from build123d import *

# Parameters (mm, degrees)
SKETCH1_W               = 31.5
SKETCH1_H               = 60
BOSS_EXTRUDE1_DEPTH     = 12.5
SKETCH2_W               = 5.015
SKETCH2_H               = 40.03
SKETCH2_W_2             = 10
CUT_EXTRUDE1_DEPTH      = 13.765
SKETCH6_R               = 3.25
CUT_EXTRUDE2_DEPTH      = 12
BOSS_EXTRUDE5_DEPTH     = 31.5
BOSS_EXTRUDE6_DEPTH     = 2
CUT_EXTRUDE3_DEPTH      = 61.634148794
CUT_EXTRUDE3_DEPTH_BACK = 61.634148794
SKETCH10_R              = 1.6


with BuildPart() as part:
    # Sketch1 → Boss-Extrude1 (new, symmetric)
    with BuildSketch(Plane(origin=(0, 0, 0), x_dir=(0, 0, -1), z_dir=(1, 0, 0))):
        with Locations((15.75, 20)):
            Rectangle(SKETCH1_W, SKETCH1_H)
    extrude(amount=BOSS_EXTRUDE1_DEPTH, both=True)

    # Sketch2 → Cut-Extrude1 (cut, symmetric)
    with BuildSketch(Plane(origin=(0, 0, -31.5), x_dir=(-1, 0, 0), z_dir=(0, 0, -1))):
        with Locations((7.5075, 20)):
            Rectangle(SKETCH2_W, SKETCH2_H)
        with Locations((0, 20)):
            Rectangle(SKETCH2_W_2, SKETCH2_H)
        with Locations((-7.5075, 20)):
            Rectangle(SKETCH2_W, SKETCH2_H)
    extrude(amount=CUT_EXTRUDE1_DEPTH, both=True, mode=Mode.SUBTRACT)

    # Sketch6 → Cut-Extrude2 (cut)
    with BuildSketch(Plane(origin=(0, 0, -31.5), x_dir=(-1, 0, 0), z_dir=(0, 0, -1))):
        with Locations(Location((-5, 44, 0), (0, 0, 90))):
            Circle(SKETCH6_R)
        with Locations(Location((5, 44, 0), (0, 0, 90))):
            Circle(SKETCH6_R)
        with Locations(Location((5, -4, 0), (0, 0, 90))):
            Circle(SKETCH6_R)
        with Locations(Location((-5, -4, 0), (0, 0, 90))):
            Circle(SKETCH6_R)
    extrude(amount=-CUT_EXTRUDE2_DEPTH, mode=Mode.SUBTRACT)

    # Sketch9 → Boss-Extrude5 (add)
    with BuildSketch(Plane(origin=(0, 0, -31.5), x_dir=(-1, 0, 0), z_dir=(0, 0, -1))):
        with BuildLine():
            Line((11.949417382, -20.681826368), (11.949417382, -24.669417382))
            Line((11.949417382, -24.669417382), (17.5, -24.669417382))
            Line((17.5, -24.669417382), (17.5, -10))
            Line((17.5, -10), (8.113106842, -10))
            ThreePointArc((8.113106842, -10), (13.410384211, -14.127322804), (11.949417382, -20.681826368))
        make_face()
        with BuildLine():
            Line((-17.5, -24.669417382), (-11.949417382, -24.669417382))
            Line((-11.949417382, -24.669417382), (-11.949417382, -20.681826368))
            ThreePointArc((-11.949417382, -20.681826368), (-13.410384211, -14.127322804), (-8.113106842, -10))
            Line((-8.113106842, -10), (-17.5, -10))
            Line((-17.5, -10), (-17.5, -24.669417382))
        make_face()
    extrude(amount=-BOSS_EXTRUDE5_DEPTH)

    # Sketch9<4> → Boss-Extrude6 (add)
    with BuildSketch(Plane(origin=(0, 0, -31.5), x_dir=(-1, 0, 0), z_dir=(0, 0, -1))):
        with BuildLine():
            Line((8.113106842, -10), (-8.113106842, -10))
            ThreePointArc((-8.113106842, -10), (-13.410384211, -14.127322804), (-11.949417382, -20.681826368))
            Line((-11.949417382, -20.681826368), (-11.949417382, -24.669417382))
            Line((-11.949417382, -24.669417382), (11.949417382, -24.669417382))
            Line((11.949417382, -24.669417382), (11.949417382, -20.681826368))
            ThreePointArc((11.949417382, -20.681826368), (13.410384211, -14.127322804), (8.113106842, -10))
        make_face()
    extrude(amount=-BOSS_EXTRUDE6_DEPTH)

    # Sketch10 → Cut-Extrude3 (cut, two sides: drawn at the far end of the back side and taken through both)
    with BuildSketch(Plane.XY.offset(-29.5).offset(-CUT_EXTRUDE3_DEPTH_BACK)):
        with Locations((-7.5, -16.25)):
            Circle(SKETCH10_R)
        with Locations((7.5, -16.25)):
            Circle(SKETCH10_R)
    extrude(amount=CUT_EXTRUDE3_DEPTH + CUT_EXTRUDE3_DEPTH_BACK, mode=Mode.SUBTRACT)


solid = part.part
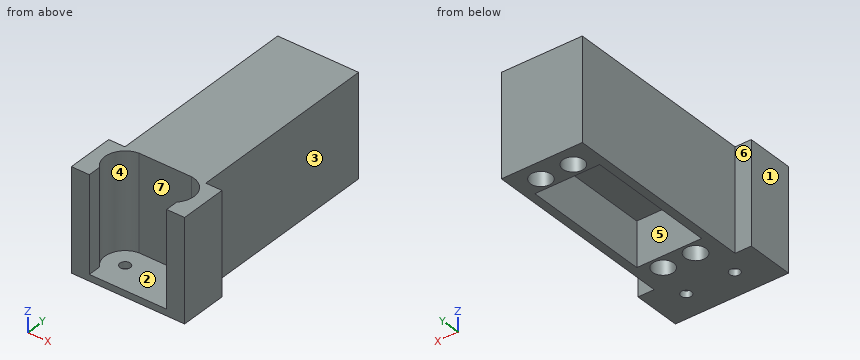
Verification items for the finished model (mm, model axes). Face numbers are marked on the shaded views. A direction names the side the tool comes from. Give positions to 0.01 mm unless a question says otherwise; leave off trailing zeros. Write each loop counter-clockwise with the first axis right and the second up, starting at its lowest first coordinate (ties: lowest second). Pieces come first, ordered by that corner, then holes. Notation, with made-up numbers: M -9,-31 L 36,-31 A23 cw 36,7 Z; hole C -28,-33.5 d8. An arc over 180 degrees is marked long. Use CSV: the item, a comma, the result in double quotes.
1) Release check for a two-part mould opening along X. For the marked faces 1, 2 and 3 record: released by +X, released by -X, zero draft, split by the parting line, or undercut.
Final values:
face 1,"released by -X"
face 2,"undercut"
face 3,"released by +X"
2) Go/stop test with flat-tipped pins: pin 1 Ø3 at (x, z) = (-7, -10) entering from -Y; pin 2 Ø8 at (y, z) = (39, -22.5) entering from +X; pin 3 Ø2.5 at (x, z) = (-16, -14.5) entering from +Y; pin 4 Ø2.5 at (x, y) = (7.5, -16.25) entering from +Z. Record where each tip stops, or that it passes through.
Final values:
pin 1,"y = -10.05"
pin 2,"x = 12.5"
pin 3,"y = -10"
pin 4,"through"
3) Cross-section at C-C (x = 5). Enter the section's corners in (y, z) (3 decimals), plus the area to 3 significant figures.
Final values:
outline,"M -24.669,-31.5 L -7.25,-31.5 L -7.25,-19.5 L -0.75,-19.5 L -0.75,-31.5 L -0.015,-31.5 L -0.015,-17.735 L 40.015,-17.735 L 40.015,-31.5 L 40.75,-31.5 L 40.75,-19.5 L 47.25,-19.5 L 47.25,-31.5 L 50,-31.5 L 50,0 L -10,0 L -10,-29.5 L -24.669,-29.5 Z"
area,"1,210 mm²"
4) Cross-section at B-B (y = -16.25). Enter the section's corners in (x, z), plus the area to 3 significant figures.
Final values:
outline,"M -17.5,-31.5 L -9.1,-31.5 L -9.1,-29.5 L -13.78,-29.5 L -13.78,0 L -17.5,0 Z; M -5.9,-31.5 L 5.9,-31.5 L 5.9,-29.5 L -5.9,-29.5 Z; M 9.1,-31.5 L 17.5,-31.5 L 17.5,0 L 13.78,0 L 13.78,-29.5 L 9.1,-29.5 Z"
area,"277 mm²"
5) Material ranges on line 1 along X through (y, z) = (44, -23); line 2 along X through (y, z) = (20.5, -23) (3 decimals); line 3 along Y through (x, z) = (15.5, -15.5), recorded low to high.
Final values:
line 1,"-12.5 to -8.25, -1.75 to 1.75, 8.25 to 12.5"
line 2,"-12.5 to -10.015, 10.015 to 12.5"
line 3,"-24.67 to -10"
6) Access from +Z, -Z, +X, -X, +Y, -Y to the whole of each face (thin tool, end or side, straight path). Record for the marked faces 4, 5, 6 and 7.
Final values:
face 4,"+Z"
face 5,"-Z"
face 6,"+Z, -Z, -X, +Y"
face 7,"+Z, -Y"
7) Cross-section at D-D (y = 26.5). Enter the section's corners in (x, z) (3 decimals), plus the area to 3 significant figures.
Final values:
outline,"M -12.5,-31.5 L -10.015,-31.5 L -10.015,-17.735 L 10.015,-17.735 L 10.015,-31.5 L 12.5,-31.5 L 12.5,0 L -12.5,0 Z"
area,"512 mm²"
8) Cross-section at A-A (z = -18.5). Enter the section's corners in (x, y) (3 decimals), plus the area to 3 significant figures.
Final values:
outline,"M -17.5,-24.669 L -11.949,-24.669 L -11.949,-20.682 A6.28 cw -8.113,-10 L 8.113,-10 A6.28 cw 11.949,-20.682 L 11.949,-24.669 L 17.5,-24.669 L 17.5,-10 L 12.5,-10 L 12.5,50 L -12.5,50 L -12.5,-10 L -17.5,-10 Z; hole M -10.015,-0.015 L 10.015,-0.015 L 10.015,40.015 L -10.015,40.015 Z"
area,"844 mm²"
